from build123d import *

# Parameters (mm, degrees)
ESBO_O1_W                = 38
ESBO_O1_H                = 12
ESBO_O1_R                = 1.7
RESSALTO_EXTRUS_O1_DEPTH = 10
FILETE1_R                = 3
ESBO_O2_R                = 8.1
CORTE_EXTRUS_O1_DEPTH    = 4
ESBO_O3_R                = 6.1
CORTE_EXTRUS_O2_DEPTH    = 5
CORTE_EXTRUS_O3_START    = -9
ESBO_O2_2_R              = 8.1
CORTE_EXTRUS_O3_DEPTH    = 4
ESBO_O4_R                = 3
CORTE_EXTRUS_O4_DEPTH    = 4


with BuildPart() as part:
    # Esboço1 → Ressalto-extrusão1 (new body)
    with BuildSketch(Plane.XY):
        Rectangle(ESBO_O1_W, ESBO_O1_H)
        with Locations((13, 0)):
            Circle(ESBO_O1_R, mode=Mode.SUBTRACT)
        with Locations((-13, 0)):
            Circle(ESBO_O1_R, mode=Mode.SUBTRACT)
    extrude(amount=RESSALTO_EXTRUS_O1_DEPTH)

    # Filete1
    filete1_edges = [part.edges().sort_by_distance(p)[0] for p in [
        (-19, -6, 5),
        (-19, 6, 5),
        (19, 6, 5),
        (19, -6, 5),
    ]]
    fillet(filete1_edges, radius=FILETE1_R)

    # Esboço2 → Corte-extrusão1 (cut)
    with BuildSketch(Plane(origin=(0, 6, 0), x_dir=(1, 0, 0), z_dir=(0, 1, 0))):
        Circle(ESBO_O2_R)
    extrude(amount=-CORTE_EXTRUS_O1_DEPTH, mode=Mode.SUBTRACT)

    # Esboço3 → Corte-extrusão2 (cut)
    with BuildSketch(Plane(origin=(0, 2, 0), x_dir=(1, 0, 0), z_dir=(0, 1, 0))):
        Circle(ESBO_O3_R)
    extrude(amount=-CORTE_EXTRUS_O2_DEPTH, mode=Mode.SUBTRACT)

    # Esboço2<2> → Corte-extrusão3 (cut)
    with BuildSketch(Plane(origin=(0, 6, 0), x_dir=(1, 0, 0), z_dir=(0, 1, 0)).offset(CORTE_EXTRUS_O3_START)):
        Circle(ESBO_O2_2_R)
    extrude(amount=-CORTE_EXTRUS_O3_DEPTH, mode=Mode.SUBTRACT)

    # Esboço4 → Corte-extrusão4 (cut)
    with BuildSketch(Plane.XY.offset(10)):
        with Locations((-13, 0)):
            Circle(ESBO_O4_R)
        with Locations((13, 0)):
            Circle(ESBO_O4_R)
    extrude(amount=-CORTE_EXTRUS_O4_DEPTH, mode=Mode.SUBTRACT)


solid = part.part
Read the model definition and answer for the solid it produces. Units are mm, in the model's axes. A direction names the side the tool comes from. Round coordinates to 2 decimals unless told otherwise and drop trailing zeros. Order: outer loops, then holes, each group sorted by start corner. A loop starts at its lowest first (then second) coordinate and runs counter-clockwise, first axis right, second up. Notation, with made-up numbers: (76, 11.25) - (85, 11.25) arc R34 ccw to (85, 43.25) - close; hole circle Ø4 at (-1, 80). An arc over 180 degrees is marked (long way). Use one line per item in the form item = value. Start each with the question number.
(1) Determine the mould class of faces 6 (the face through (11, 0, 0)), 7 (the face through (-0.2, 6, 8.3)), 8 (the face through (15, 0, 6)) for opening direction Y: +Y half, -Y half, draft (parallel to the pull), parting line (faces both ways), or undercut.
(2) The part is cut by section D-D (z = 2.25). Give the vertices of the cut face in (x, y), then the cut area to 3 significant figures.
(3) Find the intervals of material crossed by line 1 along X through (y, z) = (2.75, 7.25); line 2 along X through (y, z) = (-1.25, 2); line 3 along Y through (x, z) = (-13, 3.4), in increasing order. Write a range as from..to.
(4) The part is cut by section A-A (x = -13). Give the vertices of the cut face in (y, z), then the cut area to 3 significant figures.
(5) The part is cut by section C-C (y = 0). Give the vertices of the cut face in (x, z).
(6) Flat-ended cylindrical pins translate along their axes: pin 1 Ø2.5 at (x, z) = (2.5, 4.5) entering from -Y; pin 2 Ø1.8 at (x, y) = (-11.5, 1) entering from +Z. Find the tip coordinate at first contact, or state that the pin passes through.
(7) For faces 1 (the face through (0, 2, 6.4)), 2 (the face through (-0.2, -6, 8.3)), 3 (the face through (14.57, -0.65, 2.96)), 4 (the face through (-0.18, -4.48, 8.1)), 5 (the face through (10, 0, 8)), determine the directions among +Z, -Z, +X, -X, +Y, -Y from which every point of the face is accessible in a straight line to the end or side of a thin tool.
(8) The part is cut by section B-B (z = 9.5). Give the vertices of the cut face in (x, y), then the cut area to 3 significant figures.
Checked values:
q1.face_6 = draft
q1.face_7 = +Y half
q1.face_8 = undercut
q2.outline = (-19, -3) arc R3 ccw to (-16, -6) - (-7.78, -6) - (-7.78, -3) - (-5.67, -3) - (-5.67, 2) - (-7.78, 2) - (-7.78, 6) - (-16, 6) arc R3 ccw to (-19, 3) - close; (5.67, -3) - (7.78, -3) - (7.78, -6) - (16, -6) arc R3 ccw to (19, -3) - (19, 3) arc R3 ccw to (16, 6) - (7.78, 6) - (7.78, 2) - (5.67, 2) - close; hole circle Ø3.4 at (-13, 0); hole circle Ø3.4 at (13, 0)
q2.area = 264 mm^2
q3.line_1 = -19..-14.2, -11.8..-3.61, 3.61..11.8, 14.2..19
q3.line_2 = -19..-14.15, -11.85..-5.76, 5.76..11.85, 14.15..19
q3.line_3 = -6..-1.7, 1.7..6
q4.outline = (-6, 0) - (-1.7, 0) - (-1.7, 6) - (-3, 6) - (-3, 10) - (-6, 10) - close; (1.7, 0) - (6, 0) - (6, 10) - (3, 10) - (3, 6) - (1.7, 6) - close
q4.area = 75.6 mm^2
q5.outline = (-19, 0) - (-14.7, 0) - (-14.7, 6) - (-16, 6) - (-16, 10) - (-19, 10) - close; (-11.3, 0) - (-6.1, 0) arc R6.1 cw to (6.1, 0) - (11.3, 0) - (11.3, 6) - (10, 6) - (10, 10) - (-10, 10) - (-10, 6) - (-11.3, 6) - close; (14.7, 0) - (19, 0) - (19, 10) - (16, 10) - (16, 6) - (14.7, 6) - close
q6.pin_1 = -3
q6.pin_2 = 6
q7.face_1 = -Z, +Y
q7.face_2 = +Z, -Z, +X, -X, -Y
q7.face_3 = +Z, -Z
q7.face_4 = -Z, -Y
q7.face_5 = +Z
q8.outline = (-19, -3) arc R3 ccw to (-16, -6) - (16, -6) arc R3 ccw to (19, -3) - (19, 3) arc R3 ccw to (16, 6) - (-16, 6) arc R3 ccw to (-19, 3) - close; hole circle Ø6 at (-13, 0); hole circle Ø6 at (13, 0)
q8.area = 392 mm^2
